```python
from build123d import *

# Parameters (mm, degrees)
F0_W     = 360
F0_H     = 250
F1_DEPTH = 9
F2_W     = 320
F2_H     = 200
F3_DEPTH = 1
F4_R     = 3
F5_DEPTH = 2
F6_R     = 5
F6_R_2   = 2
F7_DEPTH = 150
F8_R     = 5
F9_R     = 1


with BuildPart() as f1:
    # F0 (on Front) → F1 (new body)
    with BuildSketch(Plane.XZ):
        with Locations((0, 125)):
            Rectangle(F0_W, F0_H)
    extrude(amount=F1_DEPTH)

    # F2 (on face) → F3 (cut)
    with BuildSketch(Plane.XZ.offset(9)):
        with Locations((0, 120)):
            Rectangle(F2_W, F2_H)
    extrude(amount=-F3_DEPTH, mode=Mode.SUBTRACT)

    # F4 (on face) → F5 (cut)
    with BuildSketch(Plane.XZ.offset(9)):
        with Locations((0, 235)):
            Circle(F4_R)
    extrude(amount=-F5_DEPTH, mode=Mode.SUBTRACT)

    # F6 (on Right) → F7 (join, symmetric)
    with BuildSketch(Plane.YZ):
        with Locations((-9, -4)):
            Circle(F6_R)
        with Locations((-9, -4)):
            Circle(F6_R_2, mode=Mode.SUBTRACT)
    extrude(amount=F7_DEPTH, both=True)

    # F8
    f8_edges = [f1.edges().sort_by_distance(p)[0] for p in [
        (180, -4.5, 0),
        (180, -4.5, 250),
        (-180, -4.5, 250),
        (-180, -4.5, 0),
    ]]
    fillet(f8_edges, radius=F8_R)

    # F9
    f9_edges = [f1.edges().sort_by_distance(p)[0] for p in [
        (-180, -9, 125),
        (-180, 0, 125),
    ]]
    fillet(f9_edges, radius=F9_R)


solid = f1.part
```
Build history of the part. All positions in model axes, mm. A direction names the side the tool comes from. Coordinates: 2 decimals unless noted, no trailing zeros. Write each loop counter-clockwise with the first axis right and the second up, starting at its lowest first coordinate (ties: lowest second). Pieces come first, ordered by that corner, then holes.
1. 3-axis set-ups, long thin cutter, end or side, ignore diameter. For faces 5 (the flat face through (-3, 0, 127)), 6 (the flat face through (-1, -9, 227)): which of +Z, -Z, +X, -X, +Y, -Y reach the whole face in a straight line?
Answer block:
face 5: +Z, -Z, +X, -X, +Y
face 6: +Z, +X, -X, -Y
2. Drop flat-ended pins along their axis: pin 1 (7.5 mm diameter, centred on x = -17.5, y = -5.5, fed in from -Z); pin 2 (3 mm diameter, centred on y = -9, z = -4, fed in from +X); pin 3 (3 mm diameter, centred on y = -10, z = -3.5, fed in from -X); pin 4 (10 mm diameter, centred on x = -47, z = 32.5, fed in from -Y). Give the stop position or say it passes through.
Answer block:
pin 1: stops at z = -9
pin 2: passes through
pin 3: stops at x = -150
pin 4: stops at y = -8
3. Drill centre lines: probe 1 along X at (y, z) = (-8, 235); probe 2 along X at (y, z) = (-8.4, 235); probe 3 along Y at (x, z) = (-137.5, 36.5). Where is each one in solid material? Low to high.
Answer block:
probe 1: x = -180 to -3, 3 to 180
probe 2: x = -179.92 to -3, 3 to 179.92
probe 3: y = -8 to 0
4. Band-saw the part on B-B, the plane z = 195. Give the cut face in (x, y), and give its area (3 significant figures).
Answer block:
outline: (-180, -8) arc R1 ccw to (-179, -9) - (-160, -9) - (-160, -8) - (160, -8) - (160, -9) - (179, -9) arc R1 ccw to (180, -8) - (180, -1) arc R1 ccw to (179, 0) - (-179, 0) arc R1 ccw to (-180, -1) - close
area: 2,920 mm2
5. Band-saw the part on A-A, the plane x = 127. Give the cut face in (y, z).
Answer block:
outline: (-9, 1) arc R5 ccw (long way) to (-6, 0) - (-1, 0) arc R1 ccw to (0, 1) - (0, 249) arc R1 ccw to (-1, 250) - (-8, 250) arc R1 ccw to (-9, 249) - (-9, 220) - (-8, 220) - (-8, 20) - (-9, 20) - close; hole circle Ø4 at (-9, -4)
6. Pull direction X, two halves, no side cores. Call faces 1 (the flat face through (-2, -4, 250)), 2 (the flat face through (180, -4, 123)), 3 (the flat face through (-180, -4, 123)), 4 (the flat face through (-2, -8, 121)): released by +X, released by -X, zero draft, split by the parting line, or undercut.
Answer block:
face 1: zero draft
face 2: released by +X
face 3: released by -X
face 4: undercut
